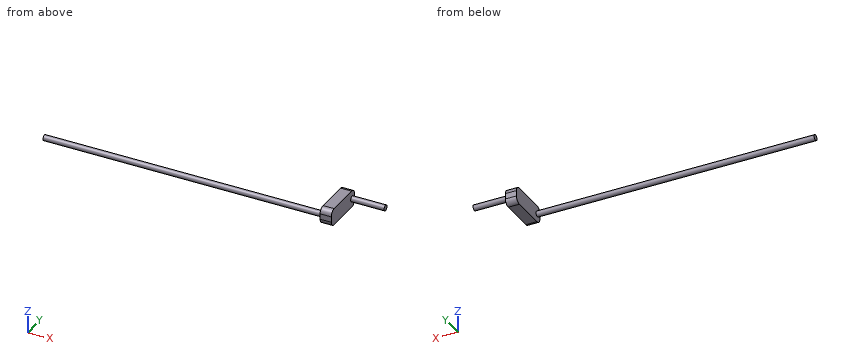
```python
from build123d import *

# Parameters (mm, degrees)
F0_W     = 40
F0_H     = 15
F0_R     = 2.5
F1_DEPTH = 10
F2_R     = 5
F3_DEPTH = 40
F4_DEPTH = 250


with BuildPart() as f1:
    # F0 (on Right) → F1 (new body)
    with BuildSketch(Plane.YZ):
        Rectangle(F0_W, F0_H)
        with Locations((-15.766867, 0)):
            Circle(F0_R, mode=Mode.SUBTRACT)
        with Locations((15.766867, 0)):
            Circle(F0_R, mode=Mode.SUBTRACT)
        with Locations((-15.766867, 0)):
            Circle(F0_R)
    extrude(amount=F1_DEPTH)

    # F2
    f2_edges = [f1.edges().sort_by_distance(p)[0] for p in [
        (5, -20, 7.5),
        (5, 20, 7.5),
        (5, -20, -7.5),
        (5, 20, -7.5),
    ]]
    fillet(f2_edges, radius=F2_R)

    # F0 (on Right) → F3 (join)
    with BuildSketch(Plane.YZ):
        with Locations((15.766867, 0)):
            Circle(F0_R)
    extrude(amount=F3_DEPTH)

    # F0 (on Right) → F4 (join)
    with BuildSketch(Plane.YZ):
        with Locations((-15.766867, 0)):
            Circle(F0_R)
    extrude(amount=-F4_DEPTH)


solid = f1.part
```
The model under review builds one solid part; all positions refer to its coordinate system, in mm. Round coordinates to 2 decimals unless told otherwise and drop trailing zeros. Write each loop counter-clockwise with the first axis right and the second up, starting at its lowest first coordinate (ties: lowest second). Pieces come first, ordered by that corner, then holes. Notation, with made-up numbers: M 8.5,14.5 L 41.5,14.5 A29 cw 41.5,49.5 Z; hole C 57,-3.5 d7. An arc over 180 degrees is marked long. Use CSV: the item, a comma, the result in double quotes. Start each with the question number.
(1) We need section A-A, the plane z = 0. State the section outline as (x, y) points.
(2) We need section C-C, the plane x = -184.5. State the section outline as (y, z) points, then the cut area to 3 significant figures.
(3) Clearance check with flat-ended pins moving along their axes: P1, Ø3, axis at x = -107.5, y = -12, coming from the +Z side; P2, Ø5, axis at x = -87.5, z = -0.5, coming from the -Y side; P3, Ø1.5, axis at y = -0.5, z = -4, coming from the +X side. State where each tip first meets the part, or that it passes through.
(4) We need section B-B, the plane y = 2. State the section outline as (x, z) points.
(5) For line 1 along X through (y, z) = (16.5, 0); line 2 along X through (y, z) = (5.5, -3.5); line 3 along Y through (x, z) = (-213, -1.5), list the stretches that pass through material, from the lowest coordinate up.
Findings:
1,outline,"M -250,-18.27 L 0,-18.27 L 0,-20 L 10,-20 L 10,13.27 L 40,13.27 L 40,18.27 L 10,18.27 L 10,20 L 0,20 L 0,-13.27 L -250,-13.27 Z"
2,outline,"C -15.77,0 d5"
2,area,"19.6 mm^2"
3,P1,"z = 1.05"
3,P2,"y = -18.27"
3,P3,"x = 10"
4,outline,"M 0,-7.5 L 10,-7.5 L 10,7.5 L 0,7.5 Z"
5,line 1,"0 to 40"
5,line 2,"0 to 10"
5,line 3,"-17.77 to -13.77"
